```python
from build123d import *

# Parameters (mm, degrees)
SKETCH_R             = 1.75
SKETCH_R_2           = 2.75
PAD_DEPTH            = 8
PAD001_DEPTH         = 20
SKETCH004_R          = 2.75
POCKET_DEPTH         = 23.001
SKETCH005_R          = 2.75
POCKET001_DEPTH      = 20.001
POCKET001_DEPTH_BACK = 8.001
SKETCH008_R          = 4
SKETCH008_R_2        = 2.75
PAD005_DEPTH         = 2
SKETCH009_R          = 3.5
SKETCH009_R_2        = 2.75
PAD006_DEPTH         = 0.55
SKETCH010_R          = 4
SKETCH010_R_2        = 2.75
PAD007_DEPTH         = 12.1
SKETCH011_R          = 3.5
SKETCH011_R_2        = 2.75
PAD008_DEPTH         = 0.55
POCKET004_DEPTH      = 2
SKETCH020_W          = 4
SKETCH020_H          = 10.5
PAD013_DEPTH         = 33.4
PAD013_DEPTH_BACK    = 23
SKETCH021_W          = 27
SKETCH021_H          = 5
PAD014_DEPTH         = 3
SKETCH029_R          = 3.75
POCKET007_DEPTH      = 1


with BuildPart() as part:
    # Sketch → Pad (new body)
    with BuildSketch(Plane.XY):
        Polygon((0, 23), (-73, 23), (-73, -3.2), (-65, -3.2), (-65, -33.4), (0, -33.4), (2, -33.4), (2, 23), align=None)
        with Locations((-23.5, 10.3)):
            Circle(SKETCH_R, mode=Mode.SUBTRACT)
        with Locations((-3.5, 10.3)):
            Circle(SKETCH_R, mode=Mode.SUBTRACT)
        with Locations((-23.5, -9.7)):
            Circle(SKETCH_R, mode=Mode.SUBTRACT)
        with Locations((-3.5, -9.7)):
            Circle(SKETCH_R, mode=Mode.SUBTRACT)
        with Locations((-55, 7)):
            Circle(SKETCH_R_2, mode=Mode.SUBTRACT)
        with Locations((-41.5, -15)):
            Circle(SKETCH_R_2, mode=Mode.SUBTRACT)
        with Locations((-54.45, -27.95)):
            Circle(SKETCH_R_2, mode=Mode.SUBTRACT)
        with Locations((-65, 7)):
            Circle(SKETCH_R_2, mode=Mode.SUBTRACT)
    extrude(amount=PAD_DEPTH)

    # Sketch001 → Pad001 (join)
    with BuildSketch(Plane(origin=(0, 0, 0), x_dir=(1, 0, 0), z_dir=(0, 0, -1))):
        Polygon((-73, -23), (-39.5, -23), (-39.5, 3.2), (-46.5, 3.2), (-57, 16.2), (-65, 16.2), (-65, 3.2), (-47.5, 3.2), (-47.5, -17), (-73, -17), align=None)
    extrude(amount=PAD001_DEPTH)

    # Sketch004 → Pocket (cut, through all)
    with BuildSketch(Plane(origin=(0, 0, 0), x_dir=(-1, 0, 0), z_dir=(0, 1, 0))):
        with Locations((55, -10)):
            Circle(SKETCH004_R)
        with Locations((65, -10)):
            Circle(SKETCH004_R)
    extrude(amount=POCKET_DEPTH, mode=Mode.SUBTRACT)

    # Sketch005 → Pocket001 (cut, two sides)
    with BuildSketch(Plane.XY) as pocket001_sk:
        with Locations((-58, -9.7)):
            Circle(SKETCH005_R)
        with Locations((-43, 7)):
            Circle(SKETCH005_R)
    extrude(amount=-POCKET001_DEPTH, mode=Mode.SUBTRACT)
    extrude(pocket001_sk.sketch, amount=POCKET001_DEPTH_BACK, mode=Mode.SUBTRACT)

    # Sketch008 → Pad005 (join)
    with BuildSketch(Plane.XY):
        with Locations((-54.45, -27.95)):
            Circle(SKETCH008_R)
        with Locations((-54.45, -27.95)):
            Circle(SKETCH008_R_2, mode=Mode.SUBTRACT)
    extrude(amount=-PAD005_DEPTH)

    # Sketch009 (on Face30 of Pad005) → Pad006 (join)
    with BuildSketch(Plane(origin=(0, 0, -2), x_dir=(1, 0, 0), z_dir=(0, 0, -1))):
        with Locations((-54.45, 27.95)):
            Circle(SKETCH009_R)
        with Locations((-54.45, 27.95)):
            Circle(SKETCH009_R_2, mode=Mode.SUBTRACT)
    extrude(amount=PAD006_DEPTH)

    # Sketch010 → Pad007 (join)
    with BuildSketch(Plane.XY):
        with Locations((-41.5, -15)):
            Circle(SKETCH010_R)
        with Locations((-41.5, -15)):
            Circle(SKETCH010_R_2, mode=Mode.SUBTRACT)
    extrude(amount=-PAD007_DEPTH)

    # Sketch011 (on Face33 of Pad007) → Pad008 (join)
    with BuildSketch(Plane(origin=(0, 0, -12.1), x_dir=(1, 0, 0), z_dir=(0, 0, -1))):
        with Locations((-41.5, 15)):
            Circle(SKETCH011_R)
        with Locations((-41.5, 15)):
            Circle(SKETCH011_R_2, mode=Mode.SUBTRACT)
    extrude(amount=PAD008_DEPTH)

    # Sketch017 (on DatumPlane) → Pocket004 (cut)
    with BuildSketch(Plane.XY.offset(8)):
        with BuildLine():
            ThreePointArc((-65, 13), (-71, 7), (-65, 1))
            Line((-65, 1), (-55, 1))
            ThreePointArc((-55, 1), (-49, 7), (-55, 13))
            Line((-55, 13), (-65, 13))
        make_face()
    extrude(amount=-POCKET004_DEPTH, mode=Mode.SUBTRACT)

    # Sketch020 → Pad013 (join, two sides)
    with BuildSketch(Plane.XZ) as pad013_sk:
        with Locations((-29, -5.25)):
            Rectangle(SKETCH020_W, SKETCH020_H)
    extrude(amount=PAD013_DEPTH)
    extrude(pad013_sk.sketch, amount=-PAD013_DEPTH_BACK)

    # Sketch021 → Pad014 (join)
    with BuildSketch(Plane(origin=(0, 0, 0), x_dir=(-1, 0, 0), z_dir=(0, 0, -1))):
        with Locations((13.5, -24.9)):
            Rectangle(SKETCH021_W, SKETCH021_H)
    extrude(amount=PAD014_DEPTH)

    # Sketch029 (on DatumPlane) → Pocket007 (cut)
    with BuildSketch(Plane.XY.offset(8)):
        with Locations((-23.5, 10.3)):
            Circle(SKETCH029_R)
        with Locations((-3.5, 10.3)):
            Circle(SKETCH029_R)
        with Locations((-23.5, -9.7)):
            Circle(SKETCH029_R)
        with Locations((-3.5, -9.7)):
            Circle(SKETCH029_R)
    extrude(amount=-POCKET007_DEPTH, mode=Mode.SUBTRACT)


solid = part.part
```
For this review, take the finished solid that the model builds, in its own axes (mm). A direction names the side the tool comes from. Round coordinates to 2 decimals unless told otherwise and drop trailing zeros. Write each loop counter-clockwise with the first axis right and the second up, starting at its lowest first coordinate (ties: lowest second). Pieces come first, ordered by that corner, then holes. Notation, with made-up numbers: (-35.75, 56) - (-27.75, 56) arc R16 ccw to (-27.75, 76) - close; hole circle Ø10 at (12.5, -19.75). An arc over 180 degrees is marked (long way). Use CSV: the item, a comma, the result in double quotes.
1) Add section B-B on z = -8.5. Write out the cut boundary in (x, y).
Conclusion:
outline,"(-73, 17) - (-67.3, 17) - (-67.3, 23) - (-73, 23) - close; (-65, -16.2) - (-57, -16.2) - (-46.5, -3.2) - (-39.5, -3.2) - (-39.5, 23) - (-52.7, 23) - (-52.7, 17) - (-47.5, 17) - (-47.5, -3.2) - (-65, -3.2) - close; (-62.7, 17) - (-57.3, 17) - (-57.3, 23) - (-62.7, 23) - close; circle Ø8 at (-41.5, -15); (-31, -33.4) - (-27, -33.4) - (-27, 23) - (-31, 23) - close; hole circle Ø5.5 at (-58, -9.7); hole circle Ø5.5 at (-43, 7); hole circle Ø5.5 at (-41.5, -15)"
2) Clearance check with flat-ended pins moving along their axes: pin 1 Ø2.5 at (x, z) = (-14.5, -2) entering from -Y; pin 2 Ø2 at (x, y) = (-5.5, 9) entering from +Z; pin 3 Ø6 at (x, y) = (-57.5, 5) entering from +Z; pin 4 Ø2.5 at (y, z) = (-24.5, -1) entering from +X. State where each tip first meets the part, or that it passes through.
Conclusion:
pin 1,"stops at y = -27.4"
pin 2,"stops at z = 7"
pin 3,"stops at z = 6"
pin 4,"stops at x = 2"
3) For faces 1 (the cylindrical face through (-71, 7, 7)), 2 (the flat face through (-39.5, 10, -10)), 3 (the flat face through (-69, -3.2, 4)), 4 (the flat face through (-13, -27.4, -1)), 5 (the cylindrical face through (-58.446, -27.774, -0.986)), list the 3-axis set-ups (+Z, -Z, +X, -X, +Y, -Y) from which the entire face can be reached by the end or side of a thin tool; tool diameter is ignored.
Conclusion:
face 1,"+Z"
face 2,"-Z, +Y"
face 3,"+Z, -Z, -X, -Y"
face 4,"-Z, +X, -Y"
face 5,"-Z"
4) Add section A-A on x = -23.5. Write out the cut boundary in (y, z).
Conclusion:
outline,"(-33.4, 0) - (-27.4, 0) - (-27.4, -3) - (-22.4, -3) - (-22.4, 0) - (-11.45, 0) - (-11.45, 7) - (-13.45, 7) - (-13.45, 8) - (-33.4, 8) - close; (-7.95, 0) - (8.55, 0) - (8.55, 7) - (6.55, 7) - (6.55, 8) - (-5.95, 8) - (-5.95, 7) - (-7.95, 7) - close; (12.05, 0) - (23, 0) - (23, 8) - (14.05, 8) - (14.05, 7) - (12.05, 7) - close"
5) The part is to be moulded in two halves that separate along X. For faces 6 (the cylindrical face through (-25.25, -9.62, 3.45)), 7 (the cylindrical face through (-3.728, 12.035, 3.451)), 8 (the flat face through (-73, 12.6, 0.4)), 9 (the flat face through (-60, 7, 0)), say which applies: pulls with the +X half, pulls with the -X half, needs draft (parallel to the pull), parting line crosses it, or undercut.
Conclusion:
face 6,"undercut"
face 7,"undercut"
face 8,"pulls with the -X half"
face 9,"needs draft"
6) Add section D-D on z = -16.25. Write out the cut boundary in (x, y), and give its area (3 significant figures).
Conclusion:
outline,"(-73, 17) - (-47.5, 17) - (-47.5, -3.2) - (-65, -3.2) - (-65, -16.2) - (-57, -16.2) - (-46.5, -3.2) - (-39.5, -3.2) - (-39.5, 23) - (-73, 23) - close; hole circle Ø5.5 at (-58, -9.7); hole circle Ø5.5 at (-43, 7)"
area,"487 mm^2"
7) Add section C-C on y = -9.7. Count the separate pieces of the cut face and the enclosed holes in it, and give its area (3 significant figures).
Conclusion:
separate pieces,"4"
enclosed holes,"0"
area,"625 mm^2"
8) Wall thickness on line 1 along X through (y, z) = (20.7, -10); line 2 along X through (y, z) = (10.3, 5.5); line 3 along Y through (x, z) = (-23.5, 3.75): over which ranges is each line inside the solid? List them lowest first. Write a range as from..to.
Conclusion:
line 1,"x = -73..-67.75, -62.25..-57.75, -52.25..-39.5, -31..-27"
line 2,"x = -73..-25.25, -21.75..-5.25, -1.75..2"
line 3,"y = -33.4..-11.45, -7.95..8.55, 12.05..23"
